```python
from build123d import *

# Parameters (mm, degrees)
F0_R      = 12.5
F2_ANGLE  = 90
F3_R      = 10
F4_DEPTH  = 10
F5_R      = 10
F8_ANGLE  = 90
F9_R      = 10
F10_DEPTH = 40
F12_ANGLE = 90
F13_R     = 10
F14_DEPTH = 28
F15_R     = 10
F15_R_2   = 5
F17_ANGLE = 20
F18_ANGLE = 45


# Not quite as in the source:
# - the program builds the solid bodies; features that only make, move or delete a surface that nothing else refers to are left out


with BuildPart() as f2:
    # F0 (on Right) → F2 (revolve)
    with BuildSketch(Plane.YZ):
        Circle(F0_R)
    revolve(axis=Axis((0, 8.0864932388, -22.5855782628), (0, 1, 0)), revolution_arc=F2_ANGLE)

    # F3 (on face) → F4 (join)
    with BuildSketch(Plane(origin=(0, 0, -22.5855782628), x_dir=(1, 0, 0), z_dir=(0, 0, -1))):
        with Locations((22.5855782628, 0)):
            Circle(F3_R)
    extrude(amount=F4_DEPTH)

    # F5 (on face) → F8 (revolve)
    with BuildSketch(Plane(origin=(0, 0, -32.5855782628), x_dir=(1, 0, 0), z_dir=(0, 0, -1))):
        with Locations((22.5855782628, 0)):
            Circle(F5_R)
    revolve(axis=Axis((45.0843572617, 2.1267626435, -32.5855782628), (0, -1, 0)), revolution_arc=F8_ANGLE)

    # F9 (on face) → F10 (join)
    with BuildSketch(Plane.YZ.offset(45.0843572617)):
        with Locations((0, -55.0843572617)):
            Circle(F9_R)
    extrude(amount=F10_DEPTH)

    # F11 (on face) → F12 (revolve)
    with BuildSketch(Plane.YZ.offset(85.0843572617)):
        with BuildLine():
            ThreePointArc((0, -45.0843572617), (-7.0710678119, -62.1554250735), (10, -55.0843572617))
            ThreePointArc((10, -55.0843572617), (7.0710678119, -48.0132894498), (0, -45.0843572617))
        make_face()
    revolve(axis=Axis((85.0843572617, 1.324259676, -40.921472013), (0, -1, 0)), revolution_arc=F12_ANGLE)

    # F13 (on face) → F14 (join)
    with BuildSketch(Plane.XY.offset(-40.921472013)):
        with Locations((99.2472425103, 0)):
            Circle(F13_R)
    extrude(amount=F14_DEPTH)

    # F15 (on face) → F17 (revolve)
    with BuildSketch(Plane.XY.offset(-12.921472013)):
        with Locations((99.2472425103, 0)):
            Circle(F15_R)
        with Locations((99.2472425103, 0)):
            Circle(F15_R_2, mode=Mode.SUBTRACT)
    revolve(axis=Axis((86.8095904589, -1.1897617951, -12.921472013), (0, -1, 0)), revolution_arc=F17_ANGLE)

    # F16 (on face) → F18 (revolve)
    with BuildSketch(Plane.XY.offset(-12.921472013)):
        with BuildLine():
            ThreePointArc((94.2472425103, 0), (99.2472425103, -5), (104.2472425103, 0))
            ThreePointArc((104.2472425103, 0), (99.2472425103, 5), (94.2472425103, 0))
        make_face()
    revolve(axis=Axis((86.8095904589, -1.1897617951, -12.921472013), (0, -1, 0)), revolution_arc=F18_ANGLE)


solid = f2.part
```
Source: CAD feature listing. Evaluate the final solid. Frame: model axes, mm. Round coordinates to 2 decimals unless told otherwise and drop trailing zeros. Write each loop counter-clockwise with the first axis right and the second up, starting at its lowest first coordinate (ties: lowest second). Pieces come first, ordered by that corner, then holes. Notation, with made-up numbers: M 14,-37 L 52,-37 A22 cw 52,-9 Z; hole C -3.5,-35 d1. An arc over 180 degrees is marked long. Answer as a JSON object with one key per item and string values. Group by question number.
(1) Ray query, line 1 (X direction, y = 5, z = -37); line 2 (X direction, y = -1, z = -48.5); line 3 (Y direction, x = 23, z = -55). Return the intervals inside material, ascending. Write a range as [from, to].
(2) Section query B-B on x = 47.5. Output: boundary loops of the cut face in (y, z).
(3) First-contact query: pin 1 (3 mm diameter, centred on x = 74.5, z = -55, fed in from -Y); pin 2 (4 mm diameter, centred on y = 2.5, z = 0.5, fed in from +X); pin 3 (3 mm diameter, centred on y = -3.5, z = -30.5, fed in from +X). Flat tips, straight axial feed; report the tip coordinate or a pass-through.
(4) Section query A-A on z = -31. Output: boundary loops of the cut face in (x, y).
(5) Mould query, pull axis X, two halves, no side actions, for faces 1 (the flat face through (95.55, 0.07, -4.18)), 2 (the flat face through (0, 0, 0)). Classes: +X half, -X half, draft (parallel to the pull), parting line (faces both ways), or undercut.
Computed values:
{
 "1": {"line 1": "[14.24, 31.97], [90.59, 107.91]", "line 2": "[16.81, 107.98]", "line 3": "[-4.43, 4.43]"},
 "2": {"outline": "C 0,-55.08 d20"},
 "3": {"pin 1": "y = -10", "pin 2": "x = 99.44", "pin 3": "x = 109.05"},
 "4": {"outline": "C 22.59,0 d20; C 99.25,0 d20"},
 "5": {"face 1": "undercut", "face 2": "-X half"}
}
